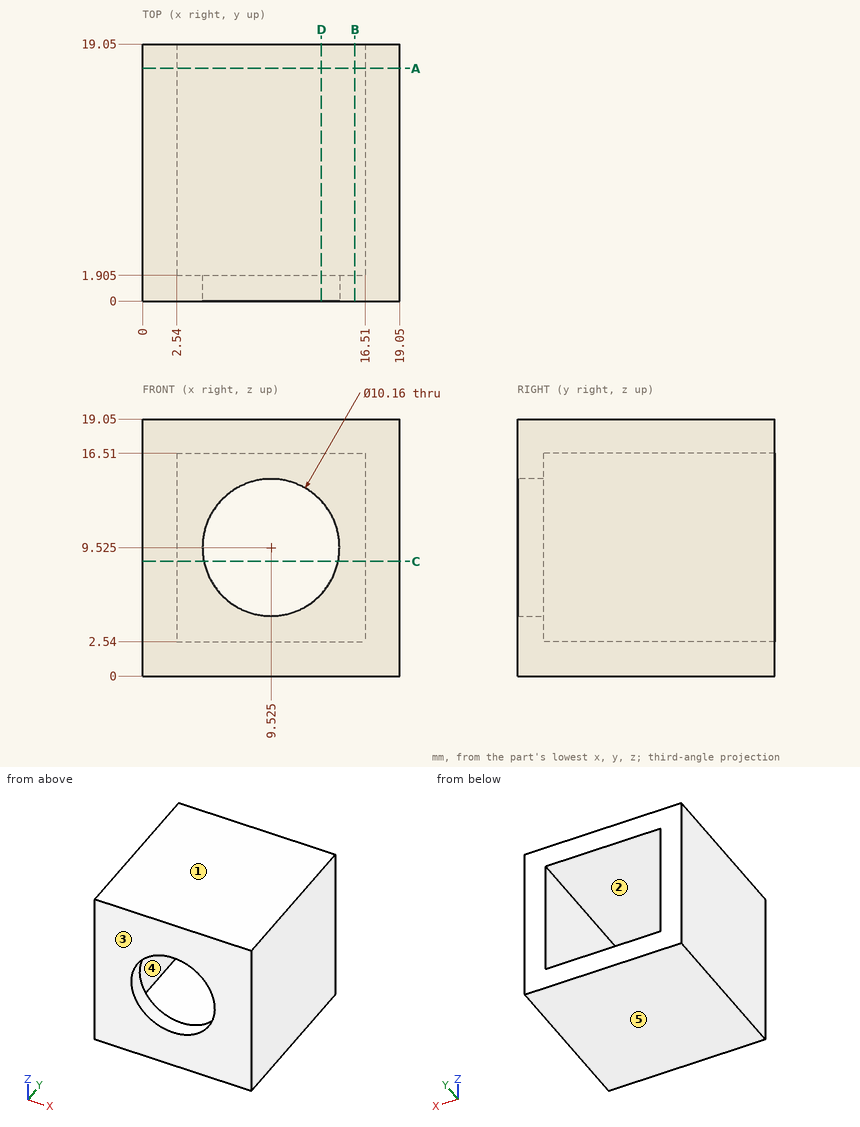
Check sheet for the drawn part. Datum: minimum x, y, z corner. Units: mm. A direction names the side the tool comes from. Coordinates: 2 decimals unless noted, no trailing zeros. Order: outer loops, then holes, each group sorted by start corner. A loop starts at its lowest first (then second) coordinate and runs counter-clockwise, first axis right, second up. Notation, with made-up numbers: (89, -28.75) - (119, -28.75) arc R21 cw to (119, -10.75) - close; hole circle Ø10 at (-22.75, 71.25). An arc over 180 degrees is marked (long way). Return JSON: item names as keys, results as strings.
(1) Section check C-C, the plane z = 8.5. Record the cut outline in (x, y) (3 decimals).
Filled sheet:
{"outline": "(0, 0) - (4.549, 0) - (4.549, 1.905) - (2.54, 1.905) - (2.54, 19.05) - (0, 19.05) - close; (14.501, 0) - (19.05, 0) - (19.05, 19.05) - (16.51, 19.05) - (16.51, 1.905) - (14.501, 1.905) - close"}
(2) Go/stop test with a flat-tipped pin: pin 1 (2 mm diameter, centred on x = 7, z = 14, fed in from +Y) (3 decimals). Record where the tip stops, or that it passes through.
Filled sheet:
{"pin 1": "stops at y = 1.905"}
(3) Section check D-D, the plane x = 13.25. Record the cut outline in (y, z) (3 decimals).
Filled sheet:
{"outline": "(0, 0) - (19.05, 0) - (19.05, 2.54) - (1.905, 2.54) - (1.905, 6.071) - (0, 6.071) - close; (0, 12.979) - (1.905, 12.979) - (1.905, 16.51) - (19.05, 16.51) - (19.05, 19.05) - (0, 19.05) - close"}
(4) Section check A-A, the plane y = 17.25. Record the cut outline in (x, z), and give its area (3 significant figures).
Filled sheet:
{"outline": "(0, 0) - (19.05, 0) - (19.05, 19.05) - (0, 19.05) - close; hole (2.54, 2.54) - (16.51, 2.54) - (16.51, 16.51) - (2.54, 16.51) - close", "area": "168 mm^2"}
(5) Mould release check, pull along Z, two halves, no side actions. Record for the marked faces 1, 2 and 3: pulls with the +Z half, pulls with the -Z half, needs draft (parallel to the pull), parting line crosses it, or undercut.
Filled sheet:
{"face 1": "pulls with the +Z half", "face 2": "undercut", "face 3": "needs draft"}
(6) Access from +Z, -Z, +X, -X, +Y, -Y to the whole of each face (thin tool, end or side, straight path). Record for the marked faces 4 and 5.
Filled sheet:
{"face 4": "+Y", "face 5": "-Z, +X, -X, +Y, -Y"}
(7) Thickness scan on line 1 along Z through (x, y) = (13.75, 8.75); line 2 along Y through (x, z) = (4.5, 16) (3 decimals). Record the ranges inside material, lowest first.
Filled sheet:
{"line 1": "z = 0 to 2.54, 16.51 to 19.05", "line 2": "y = 0 to 1.905"}
(8) Section check B-B, the plane x = 15.75. Record the cut outline in (y, z) (3 decimals), and give its area (3 significant figures).
Filled sheet:
{"outline": "(0, 0) - (19.05, 0) - (19.05, 2.54) - (1.905, 2.54) - (1.905, 16.51) - (19.05, 16.51) - (19.05, 19.05) - (0, 19.05) - close", "area": "123 mm^2"}
